Autodesk Inventor part; units mm, degrees
ref_plane "YZ Plane" through (0, 0, 0) normal (1, 0, 0) x (0, 1, 0)
ref_plane "XZ Plane" through (0, 0, 0) normal (0, 1, 0) x (-1, 0, 0)
ref_plane "XY Plane" through (0, 0, 0) normal (0, 0, 1) x (1, 0, 0)
sketch "Sketch1" plane through (0, 0, 0) normal (0, 0, 1) x (1, 0, 0)
  line L0 (9.8795, 48.1994) -> (9.8795, -53.4006)
  line L1 (16.2295, 54.5494) -> (92.4295, 54.5494)
  line L2 (98.7795, 48.1994) -> (98.7795, -53.4006)
  line L3 (22.5795, -66.1006) -> (86.0795, -66.1006)
  arc A0 (9.8795, -53.4006) -> (22.5795, -66.1006) centre (22.5795, -53.4006) ccw
  arc A1 (16.2295, 54.5494) -> (9.8795, 48.1994) centre (16.2295, 48.1994) ccw
  arc A2 (98.7795, 48.1994) -> (92.4295, 54.5494) centre (92.4295, 48.1994) ccw
  arc A3 (86.0795, -66.1006) -> (98.7795, -53.4006) centre (86.0795, -53.4006) ccw
  point P0 (0, 0)
  dimension "d0" = 12.7
  dimension "d1" = 6.35
  dimension "d2" = 120.65
  dimension "d3" = 88.9
extrude "Extrusion1" add sketch "Sketch1" along normal blind 3.175
sketch "Sketch2" plane through (0, 0, 3.175) normal (0, 0, 1) x (1, 0, 0)
  line L0 (9.8795, -53.4006) -> (9.8795, 48.1994)
  line L1 (98.7795, 48.1994) -> (98.7795, -53.4006)
  line L2 (16.2295, 54.5494) -> (92.4295, 54.5494)
  line L3 (26.6435, 49.4694) -> (82.0155, 49.4694)
  line L4 (82.0155, 49.4694) -> (82.0155, -1.3306)
  line L5 (82.0155, -1.3306) -> (26.6435, -1.3306)
  line L6 (26.6435, -1.3306) -> (26.6435, 49.4694)
  point P0 (0, 0)
  dimension "d13" = 16.764
  dimension "d14" = 16.764
  dimension "d15" = 5.08
  dimension "d16" = 55.88
extrude "Extrusion2" cut sketch "Sketch2" against normal through all
sketch "Sketch3" plane through (0, 0, 3.175) normal (0, 0, 1) x (1, 0, 0)
  line L0 (9.8795, -53.4006) -> (9.8795, 48.1994)
  line L1 (86.0795, -66.1006) -> (22.5795, -66.1006)
  line L2 (9.8795, -19.4408) -> (32.7395, -19.4408)
  line L3 (32.7395, -19.4408) -> (32.7395, -37.2208)
  line L4 (32.7395, -37.2208) -> (9.8795, -37.2208)
  point P0 (0, 0)
  dimension "d20" = 28.8798
  dimension "d21" = 46.6598
  dimension "d22" = 22.86
extrude "Extrusion3" cut sketch "Sketch3" against normal through all
sketch "Sketch4" plane through (0, 0, 3.175) normal (0, 0, 1) x (1, 0, 0)
  line L0 (9.8795, -53.4006) -> (9.8795, -37.2208)
  arc A0 (9.8795, -53.4006) -> (22.5795, -66.1006) centre (22.5795, -53.4006) ccw
  line L1 (86.0795, -66.1006) -> (22.5795, -66.1006)
  line L2 (24.8655, -43.5708) -> (24.8655, -54.1626)
  line L3 (24.8655, -43.5708) -> (9.8795, -43.5708)
  line L4 (24.8655, -54.1626) -> (9.9024, -54.1626)
  point P0 (0, 0)
  dimension "d26" = 22.5298
  dimension "d27" = 14.986
  dimension "d28" = 11.938
extrude "Extrusion4" cut sketch "Sketch4" against normal through all
sketch "Sketch5" plane through (0, 0, 3.175) normal (0, 0, 1) x (1, 0, 0)
  line L0 (86.0795, -66.1006) -> (22.5795, -66.1006)
  line L1 (9.8795, -19.4408) -> (9.8795, 48.1994)
  line L2 (9.8795, -43.5708) -> (9.8795, -37.2208)
  line L3 (28.9295, -2.1688) -> (91.1595, -2.1688)
  line L4 (91.1595, -2.1688) -> (91.1595, -11.5668)
  line L5 (91.1595, -11.5668) -> (28.9295, -11.5668)
  line L6 (28.9295, -11.5668) -> (28.9295, -2.1688)
  line L7 (28.9295, -50.4288) -> (91.1595, -50.4288)
  line L8 (91.1595, -50.4288) -> (91.1595, -59.8268)
  line L9 (91.1595, -59.8268) -> (28.9295, -59.8268)
  line L10 (28.9295, -59.8268) -> (28.9295, -50.4288)
  point P0 (0, 0)
  dimension "d31" = 54.5338
  dimension "d32" = 9.398
  dimension "d33" = 62.23
  dimension "d34" = 19.05
  dimension "d35" = 19.05
  dimension "d36" = 6.2738
extrude "Extrusion5" cut sketch "Sketch5" against normal through all
sketch "Sketch6" plane through (0, 0, 3.175) normal (0, 0, 1) x (1, 0, 0)
  line L0 (71.6015, -11.5668) -> (28.9295, -11.5668)
  line L1 (28.9295, -50.4288) -> (71.6015, -50.4288)
  line L2 (71.6015, -50.4288) -> (71.6015, -11.5668)
  line L3 (28.9295, -59.8268) -> (28.9295, -50.4288)
  line L4 (28.9295, -11.5668) -> (28.9295, -50.4288)
  line L5 (28.9295, -47.2538) -> (68.4265, -47.2538)
  line L6 (9.8795, -19.4408) -> (32.7395, -19.4408)
  line L7 (32.7395, -19.4408) -> (32.7395, -37.2208)
  line L8 (32.7395, -37.2208) -> (9.8795, -37.2208)
  line L9 (28.9295, -17.8533) -> (34.327, -17.8533)
  line L10 (34.327, -17.8533) -> (34.327, -38.8083)
  line L11 (34.327, -38.8083) -> (28.9295, -38.8083)
  line L12 (91.1595, -11.5668) -> (28.9295, -11.5668)
  line L13 (28.9295, -50.4288) -> (91.1595, -50.4288)
  line L14 (91.1595, -50.4288) -> (91.1595, -42.8088)
  line L15 (91.1595, -42.8088) -> (71.6015, -42.8088)
  line L16 (28.9295, -14.7418) -> (71.6015, -14.7418)
  line L17 (28.9295, -48.8413) -> (71.6015, -48.8413)
  line L18 (68.4265, -47.2538) -> (68.4265, -39.6338)
  line L19 (68.4265, -39.6338) -> (71.6015, -39.6338)
  line L20 (91.1595, -50.4288) -> (71.6015, -50.4288)
  line L21 (98.7795, 48.1994) -> (98.7795, -53.4006)
  line L22 (34.327, -17.8533) -> (34.327, -14.7418)
  point P0 (0, 0)
  dimension "d46" = 3.175
  dimension "d49" = 1.5875
  dimension "d50" = 1.5875
  dimension "d51" = 1.5875
  dimension "d54" = 7.62
  dimension "d55" = 3.175
  dimension "d57" = 1.5875
  dimension "d58" = 3.175
  dimension "d61" = 3.175
  dimension "d72" = 27.178
extrude "Extrusion11" cut sketch "Sketch6" against normal through all contours L2 L19 L18 L5 L4 L11 L10 L22 L16 | L15 L14 L13 L2 | L2 L1 L4 L17
sketch "Sketch7" plane through (0, 0, 3.175) normal (0, 0, 1) x (1, 0, 0)
  line L0 (71.6015, -14.7418) -> (71.6015, -39.6338)
  line L1 (71.6015, -14.7418) -> (77.9515, -14.7418)
  line L2 (77.9515, -14.7418) -> (77.9515, -39.6338)
  line L3 (77.9515, -39.6338) -> (71.6015, -39.6338)
  point P0 (0, 0)
  dimension "d64" = 6.35
extrude "Extrusion12" cut sketch "Sketch7" against normal through all
sketch "Sketch8" plane through (0, 0, 3.175) normal (0, 0, 1) x (1, 0, 0)
  line L0 (86.0795, -66.1006) -> (22.5795, -66.1006)
  line L1 (98.7795, 48.1994) -> (98.7795, -53.4006)
  line L2 (82.2695, -32.3948) -> (98.7795, -32.3948)
  line L3 (98.7795, -32.3948) -> (98.7795, -50.1748)
  line L4 (98.7795, -50.1748) -> (82.2695, -50.1748)
  line L5 (82.2695, -50.1748) -> (82.2695, -32.3948)
  point P0 (0, 0)
  dimension "d67" = 15.9258
  dimension "d68" = 17.78
  dimension "d69" = 16.51
extrude "Extrusion13" cut sketch "Sketch8" against normal through all
sketch "Sketch9" plane through (0, 0, 3.175) normal (0, 0, 1) x (1, 0, 0)
  line L0 (98.7795, 48.1994) -> (98.7795, -32.3948)
  line L1 (16.2295, 54.5494) -> (92.4295, 54.5494)
  line L2 (9.8795, -19.4408) -> (9.8795, 48.1994)
  line L3 (86.0795, -66.1006) -> (22.5795, -66.1006)
  line L4 (36.2694, 49.7107) -> (34.2897, 49.7107)
  line L5 (34.2897, 49.7107) -> (33.2998, 51.4252)
  line L6 (33.2998, 51.4252) -> (34.2897, 53.1397)
  line L7 (34.2897, 53.1397) -> (36.2694, 53.1397)
  line L8 (36.2694, 53.1397) -> (37.2593, 51.4252)
  line L9 (37.2593, 51.4252) -> (36.2694, 49.7107)
  line L10 (75.3593, 51.4252) -> (74.3694, 49.7107)
  line L11 (74.3694, 49.7107) -> (72.3897, 49.7107)
  line L12 (72.3897, 49.7107) -> (71.3998, 51.4252)
  line L13 (71.3998, 51.4252) -> (72.3897, 53.1397)
  line L14 (72.3897, 53.1397) -> (74.3694, 53.1397)
  line L15 (74.3694, 53.1397) -> (75.3593, 51.4252)
  line L16 (97.3698, 34.5095) -> (95.6553, 33.5197)
  line L17 (95.6553, 33.5197) -> (93.9408, 34.5095)
  line L18 (93.9408, 34.5095) -> (93.9408, 36.4893)
  line L19 (93.9408, 36.4893) -> (95.6553, 37.4791)
  line L20 (95.6553, 37.4791) -> (97.3698, 36.4893)
  line L21 (97.3698, 36.4893) -> (97.3698, 34.5095)
  line L22 (37.2593, -62.9764) -> (36.2694, -64.6909)
  line L23 (36.2694, -64.6909) -> (34.2897, -64.6909)
  line L24 (34.2897, -64.6909) -> (33.2998, -62.9764)
  line L25 (33.2998, -62.9764) -> (34.2897, -61.2619)
  line L26 (34.2897, -61.2619) -> (36.2694, -61.2619)
  line L27 (36.2694, -61.2619) -> (37.2593, -62.9764)
  line L28 (75.3593, -62.9764) -> (74.3694, -64.6909)
  line L29 (74.3694, -64.6909) -> (72.3897, -64.6909)
  line L30 (72.3897, -64.6909) -> (71.3998, -62.9764)
  line L31 (71.3998, -62.9764) -> (72.3897, -61.2619)
  line L32 (72.3897, -61.2619) -> (74.3694, -61.2619)
  line L33 (74.3694, -61.2619) -> (75.3593, -62.9764)
  line L34 (97.3698, -3.5905) -> (95.6553, -4.5803)
  line L35 (95.6553, -4.5803) -> (93.9408, -3.5905)
  line L36 (93.9408, -3.5905) -> (93.9408, -1.6107)
  line L37 (93.9408, -1.6107) -> (95.6553, -0.6209)
  line L38 (95.6553, -0.6209) -> (97.3698, -1.6107)
  line L39 (97.3698, -1.6107) -> (97.3698, -3.5905)
  line L40 (14.7182, 34.5095) -> (13.0037, 33.5197)
  line L41 (13.0037, 33.5197) -> (11.2892, 34.5095)
  line L42 (11.2892, 34.5095) -> (11.2892, 36.4893)
  line L43 (11.2892, 36.4893) -> (13.0037, 37.4791)
  line L44 (13.0037, 37.4791) -> (14.7182, 36.4893)
  line L45 (14.7182, 36.4893) -> (14.7182, 34.5095)
  line L46 (14.7182, -1.6107) -> (14.7182, -3.5905)
  line L47 (14.7182, -3.5905) -> (13.0037, -4.5803)
  line L48 (13.0037, -4.5803) -> (11.2892, -3.5905)
  line L49 (11.2892, -3.5905) -> (11.2892, -1.6107)
  line L50 (11.2892, -1.6107) -> (13.0037, -0.6209)
  line L51 (13.0037, -0.6209) -> (14.7182, -1.6107)
  point P0 (0, 0)
  point P1 (35.2795, 51.4252)
  point P2 (73.3795, 51.4252)
  point P3 (95.6553, 35.4994)
  point P4 (35.2795, -62.9764)
  point P5 (73.3795, -62.9764)
  point P6 (95.6553, -2.6006)
  point P7 (13.0037, 35.4994)
  point P8 (13.0037, -2.6006)
  dimension "d73" = 3.429
  dimension "d74" = 3.1242
  dimension "d75" = 3.1242
  dimension "d76" = 3.1242
  dimension "d77" = 3.1242
  dimension "d78" = 25.4
  dimension "d79" = 19.05
  dimension "d80" = 38.1
  dimension "d81" = 38.1
extrude "Extrusion14" cut sketch "Sketch9" against normal through all
sketch "Sketch10" plane through (0, 0, 0) normal (0, 0, -1) x (-1, 0, 0)
  line L0 (-11.2892, 36.4893) -> (-11.2892, 34.5095)
  line L1 (-9.8795, 48.1994) -> (-9.8795, -19.4408)
  line L2 (-26.6435, 49.4694) -> (-26.6435, -1.3306)
  line L3 (-24.1035, 32.11) -> (-24.1035, 11.79)
  line L4 (-24.1035, 32.11) -> (-9.8795, 32.11)
  line L5 (-24.1035, 11.79) -> (-9.8795, 11.79)
  point P0 (-13.0037, 33.5197)
  point P1 (0, 0)
  dimension "d84" = 2.54
  dimension "d86" = 1.4097
  dimension "d87" = 1.4097
  dimension "d88" = 20.32
extrude "Extrusion15" cut sketch "Sketch10" against normal through all
equation "\"d14\" = d13"
equation "\"d35\" = d34"
properties part number "beagle_spacer_top"
Read the model definition and answer for the solid it produces. Units are mm, in the model's axes. A direction names the side the tool comes from. Round coordinates to 2 decimals unless told otherwise and drop trailing zeros. Write each loop counter-clockwise with the first axis right and the second up, starting at its lowest first coordinate (ties: lowest second). Pieces come first, ordered by that corner, then holes. Notation, with made-up numbers: M 42,22.25 L 68,22.25 A26 cw 68,59.25 Z; hole C 74,64 d9. An arc over 180 degrees is marked long. Use a Markdown table: item, result.
1) Flat-ended cylindrical pins translate along their axes: pin 1 (1 mm diameter, centred on y = -55, z = 2, fed in from +X); pin 2 (1 mm diameter, centred on y = 24, z = 2, fed in from -X); pin 3 (1 mm diameter, centred on y = -29, z = 1, fed in from -X). Find the tip coordinate at first contact, or state that the pin passes through.
Answers follow:
| item | result |
|---|---|
| pin 1 | stops at x = 98.73 |
| pin 2 | stops at x = 24.1 |
| pin 3 | stops at x = 32.74 |
2) A tool of negligible diameter and unlimited length cuts with its end or side. For faces 5 (the flat face through (17, -54.163, 2)), 6 (the flat face through (82.016, 24, 2)), 7 (the flat face through (82.27, -38, 2)), from which of +Z, -Z, +X, -X, +Y, -Y can it reach the whole face along a straight path? Write none if from no direction.
Answers follow:
| item | result |
|---|---|
| face 5 | +Z, -Z, -X |
| face 6 | +Z, -Z |
| face 7 | +Z, -Z, +X |
3) The part is cut by section C-C (x = 19). Write down the section's boundary in (y, z) (3 decimals), plus the area to 3 significant figures.
Answers follow:
| item | result |
|---|---|
| outline | M -65.586,0 L -54.163,0 L -54.163,3.175 L -65.586,3.175 Z; M -43.571,0 L -37.221,0 L -37.221,3.175 L -43.571,3.175 Z; M -19.441,0 L 11.79,0 L 11.79,3.175 L -19.441,3.175 Z; M 32.11,0 L 54.549,0 L 54.549,3.175 L 32.11,3.175 Z |
| area | 227 mm2 |
4) The part is cut by section D-D (z = 1.3). Give the number of separate pieces and of enclosed holes in the cut face, plus the area to 3 significant figures.
Answers follow:
| item | result |
|---|---|
| separate pieces | 1 |
| enclosed holes | 11 |
| area | 3,880 mm2 |
5) For a pull along X with two mould halves and no side action, classify faces 1 (the flat face through (21, -19.441, 2)), 2 (the flat face through (91.16, -55, 2)), 3 (the flat face through (9.88, -40, 2)), 4 (the flat face through (71.602, -46, 2)) as pulls with the +X half, pulls with the -X half, needs draft (parallel to the pull), parting line crosses it, or undercut.
Answers follow:
| item | result |
|---|---|
| face 1 | needs draft |
| face 2 | undercut |
| face 3 | pulls with the -X half |
| face 4 | pulls with the +X half |
6) The part is cut by section B-B (y = 43.5). Write down the section's boundary in (x, z) (1 decimal), plus the area to 3 significant figures.
Answers follow:
| item | result |
|---|---|
| outline | M 9.9,0 L 26.6,0 L 26.6,3.2 L 9.9,3.2 Z; M 82,0 L 98.8,0 L 98.8,3.2 L 82,3.2 Z |
| area | 106 mm2 |
7) Straight lines are drawn through the part: line 1 along Y through (x, z) = (50, 1.4); line 2 along Y through (x, z) = (81.5, 2.95); line 3 along Y through (x, z) = (84.5, 1). For each, find the intervals that lie inside material, in ascending order. Write a range as [from, to].
Answers follow:
| item | result |
|---|---|
| line 1 | y = [-66.1, -59.83], [-48.84, -47.25], [-14.74, -11.57], [-2.17, -1.33], [49.47, 54.55] |
| line 2 | y = [-66.1, -59.83], [-42.81, -11.57], [-2.17, -1.33], [49.47, 54.55] |
| line 3 | y = [-66.1, -59.83], [-32.39, -11.57], [-2.17, 54.55] |
8) The part is cut by section A-A (x = 58). Write down the section's boundary in (y, z) (3 decimals), plus the area to 3 significant figures.
Answers follow:
| item | result |
|---|---|
| outline | M -66.101,0 L -59.827,0 L -59.827,3.175 L -66.101,3.175 Z; M -48.841,0 L -47.254,0 L -47.254,3.175 L -48.841,3.175 Z; M -14.742,0 L -11.567,0 L -11.567,3.175 L -14.742,3.175 Z; M -2.169,0 L -1.331,0 L -1.331,3.175 L -2.169,3.175 Z; M 49.469,0 L 54.549,0 L 54.549,3.175 L 49.469,3.175 Z |
| area | 53.8 mm2 |
